For this review, take the finished solid that the model builds, in its own axes (mm). Face numbers are marked on the shaded views. Coordinates: 2 decimals unless noted, no trailing zeros. Return JSON: item names as keys, results as strings.
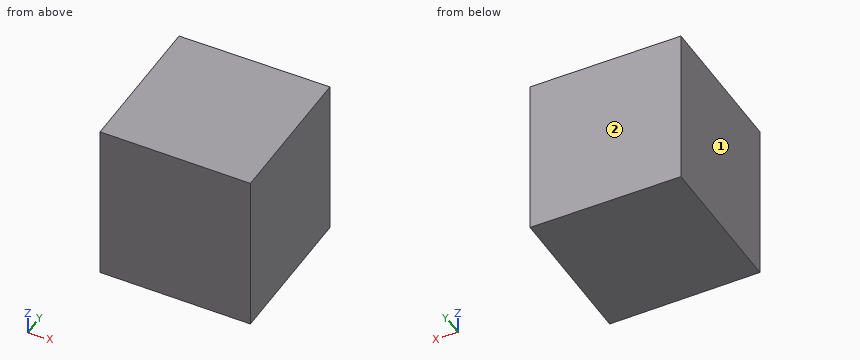
```python
from build123d import *

# Parameters (mm, degrees)
F1_DEPTH = 25.4
F2_DEPTH = 50.6288483739
F3_DEPTH = 88.0838930607


with BuildPart() as f1:
    # F0 (on Top) → F1 (new body)
    with BuildSketch(Plane.XY):
        Polygon((-76.5340924263, 75.9874135256), (-76.5340924263, -75.9874135256), (76.5340924263, -77.080771327), (76.5340924263, 75.9874135256), align=None)
    extrude(amount=F1_DEPTH)

    # F2 (add): a face of the model
    f2_faces = [f1.faces().sort_by_distance(p)[0] for p in [
        (0.0914397246, -0.2736660249, 25.4),
    ]]
    extrude(f2_faces, amount=F2_DEPTH)

    # F3 (add): a face of the model
    f3_faces = [f1.faces().sort_by_distance(p)[0] for p in [
        (0.0914397246, -0.2736660249, 0),
    ]]
    extrude(f3_faces, amount=F3_DEPTH)


solid = f1.part
```
1. Wall thickness on L1, parallel to Y at x = 1.5, z = -27; L2, parallel to Y at x = -41, z = 19.5: over which ranges is each line inside the solid? List them lowest first. Write a range as from..to.
Checks:
{"L1": "-76.54..75.99", "L2": "-76.24..75.99"}
2. Draft analysis for pull direction Y (two halves, no side actions). For the marked faces 1 and 2, state which applies: +Y half, -Y half, draft (parallel to the pull), parting line (faces both ways), or undercut.
Checks:
{"face 1": "draft", "face 2": "+Y half"}
3. Clearance check with flat-ended pins moving along their axes: pin 1 Ø1 at (x, z) = (5.5, 3) entering from -Y; pin 2 Ø10 at (x, z) = (53, -58.5) entering from -Y. State where each tip first meets the part, or that it passes through.
Checks:
{"pin 1": "y = -76.58", "pin 2": "y = -76.95"}
